The model under review builds one solid part; all positions refer to its coordinate system, in mm. Round coordinates to 2 decimals unless told otherwise and drop trailing zeros. Write each loop counter-clockwise with the first axis right and the second up, starting at its lowest first coordinate (ties: lowest second). Pieces come first, ordered by that corner, then holes.
Item 1: Add section A-A (y = 6.35). Give the boundary of the cut face in (x, z), plus the area to 3 significant figures.
Item 2: Draft analysis for pull direction X (two halves, no side actions). For faces 1 (the face through (17.53, 11.87, 3.13)), 2 (the face through (-12.24, -6.74, 3.13)), 3 (the face through (-5, -1, 0)), state which applies: +X half, -X half, draft (parallel to the pull), parting line (faces both ways), or undercut.
Item 3: Add section C-C (y = -13.5). Give the boundary of the cut face in (x, z), plus the area to 3 significant figures.
Item 4: To check wall thickness, follow L1, parallel to Y at x = 0, z = 3.25; L2, parallel to X at y = 3.5, z = 3; L3, parallel to Y at x = 4, z = 5.75. State the ranges of each line that lie inside material, in increasing order.
Item 5: Add section D-D (x = -11.5). Give the boundary of the cut face in (y, z), plus the area to 3 significant figures.
Item 6: Clearance check with flat-ended pins moving along their axes: pin 1 Ø15 at (x, y) = (11, 6.35) entering from -Z; pin 2 Ø1 at (y, z) = (0, 1) entering from +X; pin 3 Ø8.5 at (x, y) = (0, -12.7) entering from +Z; pin 4 Ø3 at (y, z) = (-15.5, 4.5) entering from +X. State where each tip first meets the part, or that it passes through.
Item 7: Add section B-B (x = 0.5). Give the boundary of the cut face in (y, z), plus the area to 3 significant figures.
```python
from build123d import *

# Parameters (mm, degrees)
F0_R     = 1.5875
F0_R_2   = 4.7625
F1_DEPTH = 6.35
F2_R     = 2.54


# Not quite as in the source:
# - a length typed as a fraction of an inch, garbled in the dataset ("3 / 203.2 mm" for 3/8 in), is restored


with BuildPart() as f1:
    # F0 (on Top) → F1 (new body)
    with BuildSketch(Plane.XY):
        Polygon((-24.1967497817, 13.97), (0, -27.94), (24.1967497817, 13.97), align=None)
        with Locations((0, -21.59)):
            Circle(F0_R, mode=Mode.SUBTRACT)
        with Locations((0, -12.7)):
            Circle(F0_R_2, mode=Mode.SUBTRACT)
        Circle(F0_R_2, mode=Mode.SUBTRACT)
        with Locations((-18.6974884677, 10.795)):
            Circle(F0_R, mode=Mode.SUBTRACT)
        with Locations((-10.9985226281, 6.35)):
            Circle(F0_R_2, mode=Mode.SUBTRACT)
        with Locations((10.9985226281, 6.35)):
            Circle(F0_R_2, mode=Mode.SUBTRACT)
        with Locations((18.6974884677, 10.795)):
            Circle(F0_R, mode=Mode.SUBTRACT)
    extrude(amount=F1_DEPTH)

    # F2
    f2_edges = [f1.edges().sort_by_distance(p)[0] for p in [
        (-24.19675, 13.97, 3.175),
        (0, -27.94, 3.175),
        (24.19675, 13.97, 3.175),
    ]]
    fillet(f2_edges, radius=F2_R)


solid = f1.part
```
Numbers:
1. outline: (-19.8, 0) - (-15.76, 0) - (-15.76, 6.35) - (-19.8, 6.35) - close; (-6.24, 0) - (6.24, 0) - (6.24, 6.35) - (-6.24, 6.35) - close; (15.76, 0) - (19.8, 0) - (19.8, 6.35) - (15.76, 6.35) - close
1. area: 130 mm2
2. face 1: undercut
2. face 2: -X half
2. face 3: draft
3. outline: (-8.34, 0) - (-4.69, 0) - (-4.69, 6.35) - (-8.34, 6.35) - close; (4.69, 0) - (8.34, 0) - (8.34, 6.35) - (4.69, 6.35) - close
3. area: 46.3 mm2
4. L1: y = -25.4 to -23.18, -20 to -17.46, -7.94 to -4.76, 4.76 to 13.97
4. L2: x = -18.15 to -14.81, -7.18 to -3.23, 3.23 to 7.18, 14.81 to 18.15
4. L3: y = -21.01 to -15.28, -10.12 to -2.58, 2.58 to 13.97
5. outline: (-8.02, 0) - (1.61, 0) - (1.61, 6.35) - (-8.02, 6.35) - close; (11.09, 0) - (13.97, 0) - (13.97, 6.35) - (11.09, 6.35) - close
5. area: 79.5 mm2
6. pin 1: stops at z = 0
6. pin 2: stops at x = 16.42
6. pin 3: passes through
6. pin 4: stops at x = 8.05
7. outline: (-25.35, 0) - (-23.1, 0) - (-23.1, 6.35) - (-25.35, 6.35) - close; (-20.08, 0) - (-17.44, 0) - (-17.44, 6.35) - (-20.08, 6.35) - close; (-7.96, 0) - (-4.74, 0) - (-4.74, 6.35) - (-7.96, 6.35) - close; (4.74, 0) - (13.97, 0) - (13.97, 6.35) - (4.74, 6.35) - close
7. area: 110 mm2
